```python
from build123d import *

# Parameters (mm, degrees)
F0_R     = 10
F1_DEPTH = 3


with BuildPart() as f1:
    # F0 (on Front) → F1 (new body)
    with BuildSketch(Plane.XZ):
        Polygon((147, -26.6665), (150, -26.6665), (150, -13.3332), (147, -13.3332), (147, 0.0001), (150, 0.0001), (150, 13.3334), (147, 13.3334), (147, 26.6667), (150, 26.6667), (150, 40), (137.5, 40), (137.5, 36.99985), (125, 36.99985), (125, 40), (112.5, 40), (112.5, 36.99985), (100, 36.99985), (100, 40), (87.5, 40), (87.5, 36.99985), (75, 36.99985), (75, 40), (62.5, 40), (62.5, 36.99985), (50, 36.99985), (50, 40), (37.5, 40), (37.5, 36.99985), (25, 36.99985), (25, 40), (12.5, 40), (12.5, 36.99985), (0, 36.99985), (0, 40), (-12.5, 40), (-12.5, 36.99985), (-25, 36.99985), (-25, 40), (-37.5, 40), (-37.5, 36.99985), (-50, 36.99985), (-50, 40), (-62.5, 40), (-62.5, 36.99985), (-75, 36.99985), (-75, 40), (-87.5, 40), (-87.5, 36.99985), (-100, 36.99985), (-100, 40), (-112.5, 40), (-112.5, 36.99985), (-125, 36.99985), (-125, 40), (-137.5, 40), (-137.5, 36.99985), (-150, 36.99985), (-150, -36.99985), (-137.5, -36.99985), (-137.5, -40), (-125, -40), (-125, -36.99985), (-112.5, -36.99985), (-112.5, -40), (-100, -40), (-100, -36.99985), (-87.5, -36.99985), (-87.5, -40), (-75, -40), (-75, -36.99985), (-62.5, -36.99985), (-62.5, -40), (-50, -40), (-50, -36.99985), (-37.5, -36.99985), (-37.5, -40), (-25, -40), (-25, -36.99985), (-12.5, -36.99985), (-12.5, -40), (0, -40), (0, -36.99985), (12.5, -36.99985), (12.5, -40), (25, -40), (25, -36.99985), (37.5, -36.99985), (37.5, -40), (50, -40), (50, -36.99985), (62.5, -36.99985), (62.5, -40), (75, -40), (75, -36.99985), (87.5, -36.99985), (87.5, -40), (100, -40), (100, -36.99985), (112.5, -36.99985), (112.5, -40), (125, -40), (125, -36.99985), (137.5, -36.99985), (137.5, -40), (147, -40), align=None)
        with Locations((85, 0)):
            Circle(F0_R, mode=Mode.SUBTRACT)
    extrude(amount=F1_DEPTH)


solid = f1.part
```
Can you work these out from the model? Positions are in its coordinate system, mm. Coordinates: 2 decimals unless noted, no trailing zeros. Write each loop counter-clockwise with the first axis right and the second up, starting at its lowest first coordinate (ties: lowest second). Pieces come first, ordered by that corner, then holes. Notation, with made-up numbers: (-37.5, -11) - (7.5, -11) arc R23 ccw to (7.5, 22) - close; hole circle Ø4 at (0.5, 56). An arc over 180 degrees is marked (long way). Return JSON: item names as keys, results as strings.
Q1. If we section it at A-A (x = 85): Please give me the cut outline in (y, z), then the cut area to 3 significant figures.
Computed values:
{"outline": "(-3, -37) - (0, -37) - (0, -10) - (-3, -10) - close; (-3, 10) - (0, 10) - (0, 37) - (-3, 37) - close", "area": "162 mm2"}
Q2. Thinking about a two-plate mould opening in X: for faces 1 (the flat face through (-2, -3, 1)), 2 (the cylindrical face through (75, -1, 0)), which applies, +X half, -X half, draft (parallel to the pull), parting line (faces both ways), or undercut?
Computed values:
{"face 1": "draft", "face 2": "undercut"}
Q3. Please list where these lines run through material, in increasing order: L1, parallel to X at y = -0.65, z = -27.5; L2, parallel to Z at x = -88.5, y = -1.25; L3, parallel to X at y = -1.8, z = 6.5. Write a range as from..to.
Computed values:
{"L1": "x = -150..147", "L2": "z = -37..37", "L3": "x = -150..77.4, 92.6..150"}
Q4. If we section it at C-C (x = -97.5): Please give me the cut outline in (y, z), then the cut area to 3 significant figures.
Computed values:
{"outline": "(-3, -37) - (0, -37) - (0, 37) - (-3, 37) - close", "area": "222 mm2"}
Q5. I'm going to push a flat-ended pin straight in: pin 1 Ø1.5 at (y, z) = (-1, -38) entering from -X. Where does the tip first touch, or does it pass through?
Computed values:
{"pin 1": "stops at x = -137.5"}
Q6. If we section it at B-B (z = -3): Please give me the cut outline in (x, y), then the cut area to 3 significant figures.
Computed values:
{"outline": "(-150, -3) - (75.46, -3) - (75.46, 0) - (-150, 0) - close; (94.54, -3) - (147, -3) - (147, 0) - (94.54, 0) - close", "area": "834 mm2"}
